from build123d import *

# Parameters (mm, degrees)
SKETCH_1_R      = 28.65
SKETCH_1_R_2    = 25.14
EXTRUDE_1_DEPTH = 5.65
SKETCH_2_R      = 27.42
SKETCH_2_R_2    = 24.94
EXTRUDE_2_DEPTH = 2.04
SKETCH_3_R      = 25
EXTRUDE_3_DEPTH = 0.5


with BuildPart() as part:
    # Эскиз1 → Бобышка-Вытянуть1 (new body)
    with BuildSketch(Plane(origin=(0, 0, 0), x_dir=(1, 0, 0), z_dir=(0, 1, 0))):
        with Locations(Location((0, 0, 0), (0, 0, 270))):
            Circle(SKETCH_1_R)
        with Locations(Location((0, 0, 0), (0, 0, 270))):
            Circle(SKETCH_1_R_2, mode=Mode.SUBTRACT)
    extrude(amount=EXTRUDE_1_DEPTH)

    # Эскиз2 → Бобышка-Вытянуть2 (add)
    with BuildSketch(Plane.XZ):
        with Locations(Location((0, 0, 0), (0, 0, 270))):
            Circle(SKETCH_2_R)
        with Locations(Location((0, 0, 0), (0, 0, 270))):
            Circle(SKETCH_2_R_2, mode=Mode.SUBTRACT)
    extrude(amount=EXTRUDE_2_DEPTH)

    # Эскиз3 → Бобышка-Вытянуть3 (add, symmetric)
    with BuildSketch(Plane(origin=(0, 0, 0), x_dir=(1, 0, 0), z_dir=(0, 1, 0))):
        with Locations(Location((0, 0, 0), (0, 0, 90))):
            Circle(SKETCH_3_R)
    extrude(amount=EXTRUDE_3_DEPTH, both=True)


solid = part.part
Geometry check sheet. Reference: the model listing, model coordinates, mm. A direction names the side the tool comes from. Give positions to 0.01 mm unless a question says otherwise; leave off trailing zeros. Order: outer loops, then holes, each group sorted by start corner. A loop starts at its lowest first (then second) coordinate and runs counter-clockwise, first axis right, second up. Notation, with made-up numbers: (50, 26.5) - (54, 26.5) arc R23 ccw to (54, 58.5) - close; hole circle Ø9 at (-12.75, -12.5). An arc over 180 degrees is marked (long way). Use one line per item in the form item = value.
1) Sectioned sample at B-B (x = 0). Record the boundary of the cut face in (y, z), and give its area (3 significant figures).
Working result:
outline = (-2.04, -27.42) - (0, -27.42) - (0, -28.65) - (5.65, -28.65) - (5.65, -25.14) - (0, -25.14) - (0, -25) - (0.5, -25) - (0.5, 25) - (0, 25) - (0, 25.14) - (5.65, 25.14) - (5.65, 28.65) - (0, 28.65) - (0, 27.42) - (-2.04, 27.42) - (-2.04, 24.94) - (-0.5, 24.94) - (-0.5, -24.94) - (-2.04, -24.94) - close
area = 99.7 mm^2
2) Sectioned sample at C-C (z = 0). Record the boundary of the cut face in (x, y), and give its area (3 significant figures).
Working result:
outline = (-28.65, 0) - (-27.42, 0) - (-27.42, -2.04) - (-24.94, -2.04) - (-24.94, -0.5) - (24.94, -0.5) - (24.94, -2.04) - (27.42, -2.04) - (27.42, 0) - (28.65, 0) - (28.65, 5.65) - (25.14, 5.65) - (25.14, 0) - (25, 0) - (25, 0.5) - (-25, 0.5) - (-25, 0) - (-25.14, 0) - (-25.14, 5.65) - (-28.65, 5.65) - close
area = 99.7 mm^2
3) Material ranges on probe 1 along X at (y, z) = (3.95, 0); probe 2 along X at (y, z) = (-1.4, 0); probe 3 along Y at (x, z) = (9, -11.5), recorded low to high. Write a range as from..to.
Working result:
probe_1 = -28.65..-25.14, 25.14..28.65
probe_2 = -27.42..-24.94, 24.94..27.42
probe_3 = -0.5..0.5
4) Draft check along Z on faces 1 (the face through (-27.5, 0, 2)), 2 (the face through (-24.542, 2.785, -5.45)), 3 (the face through (27.187, -1.006, 3.57)). Enter one of: released by +Z, released by -Z, zero draft, split by the parting line, or undercut.
Working result:
face_1 = zero draft
face_2 = undercut
face_3 = split by the parting line
5) Depth check by flat-ended pin: pin 1 Ø10 at (x, z) = (4, 19) entering from -Y; pin 2 Ø15 at (x, z) = (-5, 0) entering from +Y; pin 3 Ø3 at (x, y) = (-11.5, 4.5) entering from -Z. Enter the tip coordinate at first touch or a pass-through.
Working result:
pin_1 = -0.5
pin_2 = 0.5
pin_3 = -26.85
6) Sectioned sample at A-A (y = 2). Record the boundary of the cut face in (x, z).
Working result:
outline = circle Ø57.3 at (0, 0); hole circle Ø50.28 at (0, 0)
7) Access from +Z, -Z, +X, -X, +Y, -Y to the whole of each face (thin tool, end or side, straight path). Record for faces 4 (the face through (0, 0.5, 0)), 5 (the face through (0, -0.5, 0)), 6 (the face through (-25.3, 5.65, -0.1)).
Working result:
face_4 = +Y
face_5 = -Y
face_6 = +Z, -Z, +X, -X, +Y
